```python
from build123d import *

# Parameters (mm, degrees)
F1_DEPTH = 95
F3_DEPTH = 10.001
F4_W     = 59
F4_H     = 28
F5_DEPTH = 41.8


with BuildPart() as f1:
    # F0 (on Right) → F1 (new body)
    with BuildSketch(Plane.YZ):
        Polygon((-60, 0), (0, 0), (0, 56), (-10, 56), (-10, 28), (-60, 13), align=None)
    extrude(amount=F1_DEPTH)

    # F2 (on face) → F3 (cut, through all)
    with BuildSketch(Plane.XZ.offset(10)):
        Polygon((95, 56), (56, 56), (95, 28), align=None)
    extrude(amount=-F3_DEPTH, mode=Mode.SUBTRACT)

    # F4 (on face) → F5 (cut)
    with BuildSketch(Plane(origin=(0, 0, 0), x_dir=(1, 0, 0), z_dir=(0, 0, -1))):
        with Locations((48.5, 46)):
            Rectangle(F4_W, F4_H)
    extrude(amount=-F5_DEPTH, mode=Mode.SUBTRACT)


solid = f1.part
```
Could you check a few things on this model? Use its own coordinates, in mm. A direction names the side the tool comes from. Round coordinates to 2 decimals unless told otherwise and drop trailing zeros. Order: outer loops, then holes, each group sorted by start corner. A loop starts at its lowest first (then second) coordinate and runs counter-clockwise, first axis right, second up. Notation, with made-up numbers: M 43.5,73.5 L 51.5,73.5 A28 ccw 51.5,97.5 Z; hole C 87.5,-15.5 d2. An arc over 180 degrees is marked long. One line per question, with ' | ' between items. Start each with the question number.
(1) Suppose I cut it at D-D on z = 17.5. List the corners of the cut face in (x, y) for me.
(2) For faces 5 (the face through (75.227, -5.07, 42.196)), 6 (the face through (36, -10, 42)), 7 (the face through (19, -46, 8)), which set-ups out of +Z, -Z, +X, -X, +Y, -Y let a thin tool reach every point of the face, with its end or its side?
(3) Suppose I cut it at B-B on x = 24. List the corners of the cut face in (y, z) for me, then the cut area to 3 significant figures.
(4) For P1, Ø8.5, axis at x = 44, z = 46, coming from the -Y side; P2, Ø3, axis at x = 49.5, z = 11, coming from the -Y side; P3, Ø2, axis at y = -7, z = 33, coming from the +X side, each with a flat end and sliding along its axis, tell me the tip position at first contact or that it passes through.
(5) Suppose I cut it at C-C on y = -8.5. List the corners of the cut face in (x, z) for me, then the cut area to 3 significant figures.
(6) Thinking about a two-plate mould opening in X: for faces 1 (the face through (0, -24, 16)), 2 (the face through (48, -32, 11)), 3 (the face through (47, 0, 28)), 4 (the face through (78, -46, 8)), which applies, +X half, -X half, draft (parallel to the pull), parting line (faces both ways), or undercut?
(7) Suppose I cut it at A-A on z = 6. List the corners of the cut face in (x, y) for me.
(8) Please list where these lines run through material, in increasing order: line 1 along X through (y, z) = (-53.5, 9); line 2 along Y through (x, z) = (68, 43); line 3 along Y through (x, z) = (72.5, 20).
Geometry results:
1) outline: M 0,-45 L 19,-45 L 19,-32 L 78,-32 L 78,-45 L 95,-45 L 95,0 L 0,0 Z
2) face 5: +Z, +X, +Y, -Y | face 6: +Z, +X, -X, -Y | face 7: +Z, -Z, -Y
3) outline: M -32,0 L 0,0 L 0,56 L -10,56 L -10,28 L -32,21.4 Z | area: 1,100 mm²
4) P1: y = -10 | P2: y = -32 | P3: x = 89.43
5) outline: M 0,0 L 95,0 L 95,28 L 56,56 L 0,56 Z | area: 4,770 mm²
6) face 1: -X half | face 2: undercut | face 3: draft | face 4: undercut
7) outline: M 0,-60 L 19,-60 L 19,-32 L 78,-32 L 78,-60 L 95,-60 L 95,0 L 0,0 Z
8) line 1: 0 to 19, 78 to 95 | line 2: -10 to 0 | line 3: -32 to 0
